Geometry check sheet. Reference: the model listing, model coordinates, mm. Face numbers are marked on the shaded views. A direction names the side the tool comes from. Coordinates: 2 decimals unless noted, no trailing zeros. Loops run counter-clockwise (first coordinate to the right, second up) from the corner with the lowest first, then second, coordinate; pieces in that order, holes last. Notation, with made-up numbers: (22.25, 24.25) - (54.25, 24.25) arc R19 ccw to (54.25, 48.25) - close; hole circle Ø10 at (53.25, 21.5). An arc over 180 degrees is marked (long way). Write item = value, one per line. Start each with the question number.
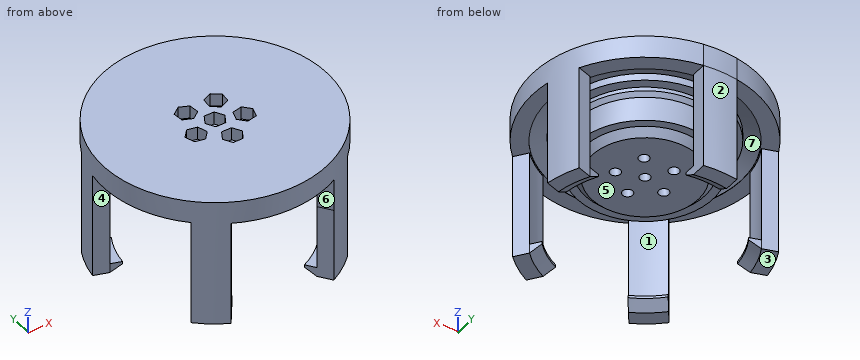
Autodesk Inventor part; units mm, degrees
ref_plane "YZ Plane" through (0, 0, 0) normal (1, 0, 0) x (0, 1, 0)
ref_plane "XZ Plane" through (0, 0, 0) normal (0, 1, 0) x (-1, 0, 0)
ref_plane "XY Plane" through (0, 0, 0) normal (0, 0, 1) x (1, 0, 0)
sketch "Эскиз1" plane through (0, 0, 0) normal (0, 0, 1) x (1, 0, 0)
  circle A0 centre (0, 0) radius 21.25
  circle A1 centre (0, 0) radius 30
  circle A2 centre (0, 0) radius 21.25
  circle A3 centre (0, 0) radius 30
  circle A4 centre (0, 0) radius 35
  line L0 (0, 0) -> (6.0777, 34.4683)
  line L1 (0, 0) -> (35, 0) construction
  line L2 (0, 0) -> (-6.0777, 34.4683)
  line L3 (0, 0) -> (35, 0) construction
  line L4 (-5.2094, 29.5442) -> (-5.2094, 34.6101)
  line L5 (5.2094, 29.5442) -> (5.2094, 34.6101)
  line L6 (-26.4884, 14.0841) -> (-31.3064, 15.6496)
  line L7 (-29.708, 4.1752) -> (-34.526, 5.7406)
  line L8 (-21.5802, -20.8398) -> (-24.5579, -24.9382)
  line L9 (-13.1511, -26.9638) -> (-16.1288, -31.0622)
  line L10 (13.1511, -26.9638) -> (16.1288, -31.0622)
  line L11 (21.5802, -20.8398) -> (24.5579, -24.9382)
  line L12 (29.708, 4.1752) -> (34.526, 5.7406)
  line L13 (26.4884, 14.0841) -> (31.3064, 15.6496)
  circle A5 centre (0, 0) radius 30.4
  point P0 (0, 0)
  point P1 (5.2094, 29.5442)
  point P2 (-5.2094, 29.5442)
  point P3 (-5.2094, 29.9503)
  point P4 (5.2094, 29.9503)
  point P5 (26.8746, 14.2096)
  point P6 (30.0943, 4.3007)
  point P7 (-30.0943, 4.3007)
  point P8 (-26.8746, 14.2096)
  point P9 (-13.3898, -27.2924)
  point P10 (-21.8189, -21.1683)
  point P11 (21.8189, -21.1683)
  point P12 (13.3898, -27.2924)
  dimension "d0" = 70
  dimension "d1" = 80
  dimension "d2" = 100
  dimension "d5" = 360
  dimension "d19" = 0.4
extrude "Выдавливание1" add sketch "Эскиз1" against normal blind 33 contours A0 L2 L0 | L0 L2 A0 | A5 L4 A4 L5 | L13 A4 L12 A5 | A5 L7 A4 L6 | A5 L9 A4 L8 | L11 A4 L10 A5
sketch "Эскиз2" plane through (0, 0, 0) normal (1, 0, 0) x (0, 1, 0)
  line L0 (30, -23) -> (30, 0)
  line L1 (-30, -19.93) -> (30, -19.93)
  line L2 (0, 0) -> (0, -33)
  line L3 (-21.25, -33) -> (21.25, -33)
  line L4 (22.45, -18.73) -> (21.25, -17.53)
  line L5 (22.45, -19.93) -> (22.45, -18.73)
  line L6 (21.25, 0) -> (21.25, -33)
  line L7 (-30, -19.93) -> (30, -19.93)
  line L8 (21.25, -2.4) -> (22.45, -1.2)
  line L9 (22.45, -1.2) -> (22.45, 0)
  line L10 (30, 0) -> (-30, 0)
  line L11 (30.4, -33) -> (30.4, 0)
  line L12 (30.4, -33) -> (30.4, 0)
  line L13 (30.4, -33) -> (30.4, 0)
  line L14 (-30, -29.93) -> (30, -29.93)
  line L15 (20.7199, -30.23) -> (27.0363, -30.23)
  line L16 (30.4, -33) -> (30.4, 0)
  line L17 (30.4, -33) -> (30.4, -30.1)
  line L18 (30.4, -33) -> (30.4, 0)
  line L19 (30.4, -30.1) -> (26.4, -30.1)
  line L20 (26.4, -30.1) -> (26.4, -30.5)
  line L21 (26.4, -30.1) -> (26.8, -30.1) construction
  line L22 (26.4, -30.5) -> (30.4, -33)
  point P0 (21.25, -19.93)
  dimension "d25" = 2.9
  dimension "d26" = 4
  dimension "d27" = 0.4
  dimension "d28" = 90
revolve "Вращение1" add sketch "Эскиз2" angle 360 about axis through (0, 0, 0) along (0, 0, -1) contours L20 L19 L11 L22 | L1 L6 L4 L5 | L9 L8 L6 L10
sketch "Эскиз3" plane through (0, 0, -33) normal (0, 0, -1) x (-1, 0, 0)
  arc A0 (5.2094, 34.6101) -> (-5.2094, 34.6101) centre (0, 0) ccw
  line L0 (-5.2094, 34.6101) -> (-5.2094, 26.4927)
  line L1 (5.2094, 34.6101) -> (5.2094, 26.4927)
  circle A1 centre (0, 0) radius 35
  line L2 (-31.3064, 15.6496) -> (-23.5862, 13.1412)
  line L3 (-34.526, 5.7406) -> (-26.8058, 3.2322)
  line L4 (-24.5579, -24.9382) -> (-19.7865, -18.371)
  line L5 (-16.1288, -31.0622) -> (-11.3575, -24.4951)
  line L6 (16.1288, -31.0622) -> (11.3575, -24.4951)
  line L7 (24.5579, -24.9382) -> (19.7865, -18.371)
  line L8 (34.526, 5.7406) -> (26.8058, 3.2322)
  line L9 (31.3064, 15.6496) -> (23.5862, 13.1412)
  circle A2 centre (0, 0) radius 27
  point P0 (0, 0)
  point P1 (5.2094, 34.6101)
  point P2 (5.2094, 34.6101)
  dimension "d13" = 360
extrude "Выдавливание2" cut sketch "Эскиз3" against normal blind 23 contours A1 L9 A2 L1 | L0 A2 L2 A1 | A2 | A1 L7 A2 L8 | L3 A2 L4 A1 | L5 A2 L6 A1
sketch "Эскиз4" plane through (0, 0, 0) normal (0, 0, 1) x (1, 0, 0)
  arc A0 (5.2094, 34.6101) -> (-5.2094, 34.6101) centre (0, 0) ccw
  circle A1 centre (0, 0) radius 35
  point P0 (0, 0)
  point P1 (5.2094, 34.6101)
extrude "Выдавливание3" add sketch "Эскиз4" along normal blind 7
sketch "Эскиз5" plane through (0, 0, 0) normal (1, 0, 0) x (0, 1, 0)
  line L0 (-21.25, -10) -> (21.25, -10)
  line L1 (21.25, -10) -> (-21.25, -10)
  line L2 (21.25, -10) -> (18.75, -10)
  line L3 (18.75, -10) -> (16.6287, -12.1213)
  line L4 (16.6287, -12.1213) -> (0, -12.1213)
  line L5 (14.2096, 0) -> (14.2096, -30.1)
  line L6 (0, -12.1213) -> (0, -10)
  point P0 (0, 0)
  dimension "d29" = 2.5
  dimension "d30" = 3
  dimension "d31" = 135
revolve "Вращение2" add sketch "Эскиз5" angle 360 about axis through (0, 0, -12.1213) along (0, 0, 1)
sketch "Эскиз6" plane through (0, 0, 0) normal (1, 0, 0) x (0, 1, 0)
  line L0 (25.52, -29.93) -> (25.52, 0)
  line L1 (25.52, 0) -> (25.52, 2)
  line L2 (30.4, -30.1) -> (30.4, 0)
  line L3 (29.9503, 0) -> (29.9503, -30.1)
  line L4 (25.52, 2) -> (29.9503, 0)
  line L5 (30.1003, -30.1) -> (30.1003, 0.0969)
  line L6 (30.1003, 0.0969) -> (25.37, 2.2323)
  line L7 (25.37, 2.2323) -> (25.37, 0)
  line L8 (25.37, 0) -> (25.37, -29.93)
  line L9 (35, 7) -> (-35, 7)
  line L10 (0, 7) -> (0, 0)
  line L11 (25.37, 0) -> (30.3149, 0)
  line L12 (34.6101, 0) -> (15.6496, 0)
  point P0 (30.1003, 0)
  dimension "d33" = 0.15
revolve "Вращение3" cut sketch "Эскиз6" angle 360 about axis through (0, 0, 7) along (0, 0, -1)
sketch "Эскиз7" plane through (0, 0, -12.1213) normal (0, 0, -1) x (-1, 0, 0)
  line L0 (15.0382, 14.3621) -> (21.6953, 20.7199)
  arc A0 (21.6953, 20.7199) -> (13.0016, 27.0363) centre (0, 0) ccw
  line L1 (13.0016, 27.0363) -> (9.0121, 18.7403)
  arc A1 (-9.0121, 18.7403) -> (9.0121, 18.7403) centre (0, 23.0741) ccw
  line L2 (-9.0121, 18.7403) -> (-13.0016, 27.0363)
  arc A2 (-13.0016, 27.0363) -> (-21.6953, 20.7199) centre (0, 0) ccw
  line L3 (-21.6953, 20.7199) -> (-15.0382, 14.3621)
  arc A3 (-20.608, -2.7799) -> (-15.0382, 14.3621) centre (-21.9448, 7.1303) ccw
  line L4 (-20.608, -2.7799) -> (-29.7307, -4.0106)
  arc A4 (-29.7307, -4.0106) -> (-26.41, -14.2307) centre (0, 0) ccw
  line L5 (-26.41, -14.2307) -> (-18.3062, -9.864)
  arc A5 (-3.7243, -20.4584) -> (-18.3062, -9.864) centre (-13.5626, -18.6674) ccw
  line L6 (-3.7243, -20.4584) -> (-5.373, -29.5149)
  arc A6 (-5.373, -29.5149) -> (5.373, -29.5149) centre (0, 0) ccw
  line L7 (5.373, -29.5149) -> (3.7243, -20.4584)
  arc A7 (18.3062, -9.864) -> (3.7243, -20.4584) centre (13.5626, -18.6674) ccw
  line L8 (18.3062, -9.864) -> (26.41, -14.2307)
  arc A8 (26.41, -14.2307) -> (29.7307, -4.0106) centre (0, 0) ccw
  line L9 (29.7307, -4.0106) -> (20.608, -2.7799)
  arc A9 (15.0382, 14.3621) -> (20.608, -2.7799) centre (21.9448, 7.1303) ccw
  circle A10 centre (-4.7023, 6.4721) radius 1.6
  circle A11 centre (0, 0) radius 1.6
  circle A12 centre (0, -8) radius 1.6
  circle A13 centre (4.7023, 6.4721) radius 1.6
  circle A14 centre (7.6085, -2.4721) radius 1.6
  circle A15 centre (-7.6085, -2.4721) radius 1.6
  line L10 (15.0382, 14.3621) -> (21.6953, 20.7199)
  arc A16 (21.6953, 20.7199) -> (13.0016, 27.0363) centre (0, 0) ccw
  line L11 (13.0016, 27.0363) -> (9.0121, 18.7403)
  arc A17 (-9.0121, 18.7403) -> (9.0121, 18.7403) centre (0, 23.0741) ccw
  line L12 (-9.0121, 18.7403) -> (-13.0016, 27.0363)
  arc A18 (-13.0016, 27.0363) -> (-21.6953, 20.7199) centre (0, 0) ccw
  line L13 (-21.6953, 20.7199) -> (-15.0382, 14.3621)
  arc A19 (-20.608, -2.7799) -> (-15.0382, 14.3621) centre (-21.9448, 7.1303) ccw
  line L14 (-20.608, -2.7799) -> (-29.7307, -4.0106)
  arc A20 (-29.7307, -4.0106) -> (-26.41, -14.2307) centre (0, 0) ccw
  line L15 (-26.41, -14.2307) -> (-18.3062, -9.864)
  arc A21 (-3.7243, -20.4584) -> (-18.3062, -9.864) centre (-13.5626, -18.6674) ccw
  line L16 (-3.7243, -20.4584) -> (-5.373, -29.5149)
  arc A22 (-5.373, -29.5149) -> (5.373, -29.5149) centre (0, 0) ccw
  line L17 (5.373, -29.5149) -> (3.7243, -20.4584)
  arc A23 (18.3062, -9.864) -> (3.7243, -20.4584) centre (13.5626, -18.6674) ccw
  line L18 (18.3062, -9.864) -> (26.41, -14.2307)
  arc A24 (26.41, -14.2307) -> (29.7307, -4.0106) centre (0, 0) ccw
  line L19 (29.7307, -4.0106) -> (20.608, -2.7799)
  arc A25 (15.0382, 14.3621) -> (20.608, -2.7799) centre (21.9448, 7.1303) ccw
  point P0 (0, 0)
extrude "Выдавливание4" cut sketch "Эскиз7" against normal up to surface (19.1213 mm away) contours A10 | A11 | A12 | A13 | A14 | A15
sketch "Эскиз8" plane through (0, 0, 7) normal (0, 0, 1) x (1, 0, 0)
  circle A0 centre (0, 0) radius 1.6
  line L0 (0, 0) -> (0, 2.7)
  circle A1 centre (0, -8) radius 1.6
  line L1 (0, -8) -> (0, -5.3)
  line L2 (1.5588, -5.3) -> (3.1177, -8)
  line L3 (3.1177, -8) -> (1.5588, -10.7)
  line L4 (1.5588, -10.7) -> (-1.5588, -10.7)
  line L5 (-1.5588, -10.7) -> (-3.1177, -8)
  line L6 (-3.1177, -8) -> (-1.5588, -5.3)
  line L7 (-1.5588, -5.3) -> (1.5588, -5.3)
  line L8 (1.5588, 2.7) -> (3.1177, 0)
  line L9 (3.1177, 0) -> (1.5588, -2.7)
  line L10 (1.5588, -2.7) -> (-1.5588, -2.7)
  line L11 (-1.5588, -2.7) -> (-3.1177, 0)
  line L12 (-3.1177, 0) -> (-1.5588, 2.7)
  line L13 (-1.5588, 2.7) -> (1.5588, 2.7)
  line L14 (4.5589, -3.1203) -> (5.5223, -0.1552)
  line L15 (7.6085, -2.4721) -> (5.0406, -1.6378)
  line L16 (6.645, -5.4372) -> (4.5589, -3.1203)
  line L17 (9.6946, -4.789) -> (6.645, -5.4372)
  line L18 (10.658, -1.8239) -> (9.6946, -4.789)
  line L19 (8.5719, 0.493) -> (10.658, -1.8239)
  line L20 (5.5223, -0.1552) -> (8.5719, 0.493)
  line L21 (4.3764, 3.3715) -> (1.8541, 5.2041)
  line L22 (4.7023, 6.4721) -> (3.1153, 4.2878)
  line L23 (7.2245, 4.6396) -> (4.3764, 3.3715)
  line L24 (7.5504, 7.7402) -> (7.2245, 4.6396)
  line L25 (5.0282, 9.5727) -> (7.5504, 7.7402)
  line L26 (2.18, 8.3047) -> (5.0282, 9.5727)
  line L27 (1.8541, 5.2041) -> (2.18, 8.3047)
  line L28 (-1.8541, 5.2041) -> (-4.3764, 3.3715)
  line L29 (-4.7023, 6.4721) -> (-3.1153, 4.2878)
  line L30 (-2.18, 8.3047) -> (-1.8541, 5.2041)
  line L31 (-5.0282, 9.5727) -> (-2.18, 8.3047)
  line L32 (-7.5504, 7.7402) -> (-5.0282, 9.5727)
  line L33 (-7.2245, 4.6396) -> (-7.5504, 7.7402)
  line L34 (-4.3764, 3.3715) -> (-7.2245, 4.6396)
  line L35 (-5.5223, -0.1552) -> (-4.5589, -3.1203)
  line L36 (-7.6085, -2.4721) -> (-5.0406, -1.6378)
  line L37 (-8.5719, 0.493) -> (-5.5223, -0.1552)
  line L38 (-10.658, -1.8239) -> (-8.5719, 0.493)
  line L39 (-9.6946, -4.789) -> (-10.658, -1.8239)
  line L40 (-6.645, -5.4372) -> (-9.6946, -4.789)
  line L41 (-4.5589, -3.1203) -> (-6.645, -5.4372)
  point P0 (0, 0)
  dimension "d40" = 2.7
  dimension "d41" = 2.7
  dimension "d44" = 360
extrude "Выдавливание5" cut sketch "Эскиз8" against normal blind 4
properties part number "tire disk"
(1) Draft check along Z on the marked faces 1, 2 and 3. Enter one of: pulls with the +Z half, pulls with the -Z half, needs draft (parallel to the pull), parting line crosses it, or undercut.
(2) Sectioned sample at B-B on z = -25. Enter the section's corners in (x, y), plus the area to 3 significant figures.
(3) Depth check by flat-ended pin: pin 1 (1.5 mm diameter, centred on y = -28, z = -27, fed in from +X); pin 2 (5 mm diameter, centred on x = 0, y = 0, fed in from -Z); pin 3 (6 mm diameter, centred on x = 25.5, y = 24, fed in from -Z); pin 4 (2.5 mm diameter, centred on x = -1, y = -6.5, fed in from +Z). Enter the tip coordinate at first touch or a pass-through.
(4) Sectioned sample at A-A on z = -8. Count the separate pieces of the cut face and the enclosed holes in it, plus the area to 3 significant figures.
(5) Tool access check on the marked faces 4, 5, 6 and 7. Record the directions out of +Z, -Z, +X, -X, +Y, -Y that give a thin tool (end or side, any length) a straight path to the whole face; none if there is none.
(6) Scan lines: line 1 (Y direction, x = -9, z = 2); line 2 (Z direction, x = 3.5, y = 12); line 3 (Z direction, x = -7, y = -31.5). Record each from-to range of solid material in increasing order.
Working result:
q1.face_1 = undercut
q1.face_2 = needs draft
q1.face_3 = pulls with the -Z half
q2.outline = (-34.53, 5.74) - (-30.09, 4.3) arc R30.4 cw to (-26.87, 14.21) - (-31.31, 15.65) arc R35 ccw to start; (-24.56, -24.94) arc R35 ccw to (-16.13, -31.06) - (-13.39, -27.29) arc R30.4 cw to (-21.82, -21.17) - close; (-5.21, 29.95) arc R30.4 cw to (5.21, 29.95) - (5.21, 34.61) arc R35 ccw to (-5.21, 34.61) - close; (13.39, -27.29) - (16.13, -31.06) arc R35 ccw to (24.56, -24.94) - (21.82, -21.17) arc R30.4 cw to start; (26.87, 14.21) arc R30.4 cw to (30.09, 4.3) - (34.53, 5.74) arc R35 ccw to (31.31, 15.65) - close
q2.area = 241 mm2
q3.pin_1 = 21.96
q3.pin_2 = -12.12
q3.pin_3 = 0
q3.pin_4 = 7
q4.separate_pieces = 6
q4.enclosed_holes = 6
q4.area = 1,610 mm2
q5.face_4 = -Z, -X, -Y
q5.face_5 = -Z
q5.face_6 = -Z, -Y
q5.face_7 = none
q6.line_1 = -33.82 to -24.27, -23.72 to -3.26, -1.68 to 23.72, 24.27 to 33.82
q6.line_2 = -12.12 to 7
q6.line_3 = 0 to 7
